Autodesk Inventor part; units mm, degrees
ref_plane "YZ Plane" through (0, 0, 0) normal (1, 0, 0) x (0, 1, 0)
ref_plane "XZ Plane" through (0, 0, 0) normal (0, 1, 0) x (-1, 0, 0)
ref_plane "XY Plane" through (0, 0, 0) normal (0, 0, 1) x (1, 0, 0)
sketch "Sketch1" plane through (0, 0, 0) normal (0, 1, 0) x (-1, 0, 0)
  circle A0 centre (0, 0) radius 30
  dimension "d0" = 60
extrude "Extrusion1" add sketch "Sketch1" along normal blind 2.5
sketch "Sketch2" plane through (0, 2.5, 0) normal (0, 1, 0) x (1, 0, 0)
  circle A0 centre (0, 0) radius 30
  circle A1 centre (0, 0) radius 27
  circle A2 centre (0, 0) radius 30 construction
  line L0 (-28.6529, -8.8889) -> (-25.7876, -8)
  line L1 (-25.7876, 8) -> (-28.6529, 8.8889)
  line L2 (-25.7876, -8) -> (-25.7876, 8) construction
  arc A3 (-28.6529, 8.8889) -> (-28.6529, -8.8889) centre (0, 0) ccw
  arc A4 (-25.7876, 8) -> (-25.7876, -8) centre (0, 0) ccw
  dimension "d3" = 3
  dimension "d4" = 16
extrude "Extrusion2" add sketch "Sketch2" along normal blind 6 contours L1 A1 L0 A0 picked at (-28.0966, 6.6307)
fillet "Fillet1" radius 2 2 edges at (-25.7876, 5.5, 8) (-25.7876, 5.5, -8)
pattern_circular "Circular Pattern1" count 4 over 360 about axis through (0, 0, 0) along (0, 1, 0) of "Fillet1", "Extrusion2"
sketch "Sketch3" plane through (0, 0, 0) normal (0, -1, 0) x (1, 0, 0)
  circle A0 centre (0, 0) radius 17
  dimension "d11" = 34
extrude "Extrusion3" cut sketch "Sketch3" against normal through all
properties part number "button_barrel" material "ABS Plastic"
Could you check a few things on this model? Use its own coordinates, in mm. A direction names the side the tool comes from. Give positions to 0.01 mm unless a question says otherwise; leave off trailing zeros. Write each loop counter-clockwise with the first axis right and the second up, starting at its lowest first coordinate (ties: lowest second). Pieces come first, ordered by that corner, then holes. Notation, with made-up numbers: (-21, 58) - (-3, 58) arc R22 cw to (-3, 91) - close; hole circle Ø11 at (65, 27.25). An arc over 180 degrees is marked (long way). Use CSV: the item, a comma, the result in double quotes. Start each with the question number.
Item 1: I'm going to push flat-ended pins straight in: pin 1 (1.5 mm diameter, centred on x = 15.5, z = 4.5, fed in from -Y); pin 2 (3 mm diameter, centred on y = 2, z = -12.5, fed in from -X); pin 3 (5 mm diameter, centred on x = -19.5, y = 2.5, fed in from -Z). Where does each tip first touch, or does it pass through?
Item 2: For faces 1 (the face through (27, 5, 0)), 2 (the face through (-28, 8.5, 0)), which set-ups out of +Z, -Z, +X, -X, +Y, -Y let a thin tool reach every point of the face, with its end or its side?
Item 3: I want a section at B-B, the plane z = 16. Please give me the cut outline in (x, y).
Item 4: If we mould it in two halves opening along X, with no side actions, what happens to faces 3 (the face through (-27, 5, 0)), 4 (the face through (-2.66, 3.25, -29.88)), 5 (the face through (0, 8.5, -28))? For each: pulls with the +X half, pulls with the -X half, needs draft (parallel to the pull), parting line crosses it, or undercut.
Item 5: I want a section at D-D, the plane y = 0.75. Please give me the cut outline in (x, z).
Item 6: I want a section at A-A, the plane x = 0. Please give me the cut outline in (y, z).
Item 7: I want a section at C-C, the plane y = 4. Please give me the cut outline in (x, z), then the cut area to 3 significant figures.
Item 8: If I drill on line 1 along Z through (x, y) = (0, 0.75); line 2 along X through (y, z) = (7.5, 0.5); line 3 along Y through (x, z) = (7, 22), over which ranges is the centre line in solid material (lowest first)?
Findings:
1,pin 1,"passes through"
1,pin 2,"stops at x = -27.91"
1,pin 3,"stops at z = -24.72"
2,face 1,"+Y"
2,face 2,"+Z, -Z, +X, -X, +Y"
3,outline,"(-25.38, 0) - (-5.74, 0) - (-5.74, 2.5) - (-25.38, 2.5) - close; (5.74, 0) - (25.38, 0) - (25.38, 2.5) - (5.74, 2.5) - close"
4,face 3,"undercut"
4,face 4,"parting line crosses it"
4,face 5,"needs draft"
5,outline,"circle Ø60 at (0, 0); hole circle Ø34 at (0, 0)"
6,outline,"(0, -30) - (8.5, -30) - (8.5, -27) - (2.5, -27) - (2.5, -17) - (0, -17) - close; (0, 17) - (2.5, 17) - (2.5, 27) - (8.5, 27) - (8.5, 30) - (0, 30) - close"
7,outline,"(-28.65, -8.89) - (-27.63, -8.57) arc R2 ccw to (-26.28, -6.2) arc R27 cw to (-26.28, 6.2) arc R2 ccw to (-27.63, 8.57) - (-28.65, 8.89) arc R30 ccw to start; (-8.89, -28.65) arc R30 ccw to (8.89, -28.65) - (8.57, -27.63) arc R2 ccw to (6.2, -26.28) arc R27 cw to (-6.2, -26.28) arc R2 ccw to (-8.57, -27.63) - close; (-8.89, 28.65) - (-8.57, 27.63) arc R2 ccw to (-6.2, 26.28) arc R27 cw to (6.2, 26.28) arc R2 ccw to (8.57, 27.63) - (8.89, 28.65) arc R30 ccw to start; (26.28, -6.2) arc R2 ccw to (27.63, -8.57) - (28.65, -8.89) arc R30 ccw to (28.65, 8.89) - (27.63, 8.57) arc R2 ccw to (26.28, 6.2) arc R27 cw to start"
7,area,"200 mm2"
8,line 1,"z = -30 to -17, 17 to 30"
8,line 2,"x = -30 to -27, 27 to 30"
8,line 3,"y = 0 to 2.5"
